```python
from build123d import *

# Parameters (mm, degrees)
F0_W            = 304.8
F0_H            = 203.2
F1_DEPTH        = 19.05
F2_W            = 228.6
F2_H            = 25.4
F3_DEPTH        = 19.051
F5_D            = 6.35
F6_R            = 6.35
F8_D            = 12.7
F9_R            = 5.4271203762
F9_R_2          = 6.35
F10_DEPTH       = 12.7
F12_D           = 9.525
F12_CBORE_D     = 15.875
F12_CBORE_DEPTH = 12.7
F13_SIZE        = 50.8


with BuildPart() as f1:
    # F0 (on Front) → F1 (new body)
    with BuildSketch(Plane.XZ):
        with Locations((152.4, 101.6)):
            Rectangle(F0_W, F0_H)
    extrude(amount=F1_DEPTH)

    # F2 (on face) → F3 (cut, through all)
    with BuildSketch(Plane.XZ.offset(19.05)):
        with Locations((152.4, 12.7)):
            Rectangle(F2_W, F2_H)
    extrude(amount=-F3_DEPTH, mode=Mode.SUBTRACT)

    # F5 (through all)
    with Locations(Plane.XZ.offset(19.05)):
        with Locations((120.65, 38.1), (184.15, 38.1)):
            Hole(F5_D / 2)

    # F6
    f6_edges = [f1.edges().sort_by_distance(p)[0] for p in [
        (38.1, -9.525, 0),
        (38.1, -9.525, 25.4),
        (0, -9.525, 0),
        (266.7, -9.525, 25.4),
        (266.7, -9.525, 0),
        (304.8, -9.525, 0),
    ]]
    fillet(f6_edges, radius=F6_R)

    # F8 (through all)
    with Locations(Plane.XZ.offset(19.05)):
        with Locations((152.4, 105.6132)):
            Hole(F8_D / 2)

    # F9 (on face) → F10 (cut)
    with BuildSketch(Plane(origin=(0, 0, 0), x_dir=(-1, 0, 0), z_dir=(0, 1, 0))):
        with Locations((-25.4, 137.3632)):
            Circle(F9_R)
        with Locations((-279.4, 137.3632)):
            Circle(F9_R_2)
    extrude(amount=-F10_DEPTH, mode=Mode.SUBTRACT)

    # F12 (through all)
    with Locations(Plane(origin=(0, 0, 0), x_dir=(-1, 0, 0), z_dir=(0, 1, 0))):
        with Locations((-286.227653817, 94.6363272378), (-285.75, 18.4363272378), (-19.05, 18.4363272378), (-16.3299310523, 94.6363272378)):
            CounterBoreHole(F12_D / 2, F12_CBORE_D / 2, F12_CBORE_DEPTH)

    # F13
    f13_edges = [f1.edges().sort_by_distance(p)[0] for p in [
        (304.8, -9.525, 203.2),
        (0, -9.525, 203.2),
    ]]
    chamfer(f13_edges, length=F13_SIZE)


solid = f1.part
```
Part model, mm, in its own coordinate system. A direction names the side the tool comes from. Round coordinates to 2 decimals unless told otherwise and drop trailing zeros. Order: outer loops, then holes, each group sorted by start corner. A loop starts at its lowest first (then second) coordinate and runs counter-clockwise, first axis right, second up. Notation, with made-up numbers: M 79.25,79.5 L 131.25,79.5 A9 cw 131.25,96.5 Z; hole C 82,53.5 d7. An arc over 180 degrees is marked long. Answer in a Markdown table with one row per item. Add a question column.
Q1. Pin check, flat tips, straight feed: pin 1 (1 mm diameter, centred on x = 271.5, y = -9, fed in from +Z); pin 2 (12.5 mm diameter, centred on x = 19.05, z = 18.44, fed in from +Y); pin 3 (2 mm diameter, centred on x = 263, y = -4, fed in from +Z). Stop position of each tip, or through.
Q2. Cut at B-B on x = 120.65. Give the cut face in (y, z) (3 decimals).
Q3. Mould opens along Z. For faces 4 (the face through (19, -12.7, 13)), 5 (the face through (288.79, -15.92, 98.65)), 6 (the face through (304.8, -9, 78)), 7 (the face through (151, -10, 25.4)) say: +Z half, -Z half, draft (parallel to the pull), parting line (faces both ways), or undercut.
Q4. Wall check: L1, parallel to X at y = -4.75, z = 90; L2, parallel to Y at x = 290, z = 88; L3, parallel to Z at x = 70, y = -13.75. Give the ranges that are in metal, low to high. Write a range as from..to.
Q5. Cut at A-A on z = 38.1. Give the cut face in (x, y) (3 decimals), and give its area (3 significant figures).
Q6. Cut at C-C on y = -9.5. Give the number of separate pieces and of enclosed holes in the cut face, and give its area (3 significant figures).
Q7. 3-axis set-ups, long thin cutter, end or side, ignore diameter. For faces 1 (the face through (150, 0, 126)), 2 (the face through (279, -12.7, 137)), 3 (the face through (264.79, -9.39, 23.59)): which of +Z, -Z, +X, -X, +Y, -Y reach the whole face in a straight line?
Q8. Cut at D-D on x = 78.5. Give the cut face in (y, z).
Established:
| question | item | result |
|---|---|---|
| 1 | pin 1 | stops at z = 186.2 |
| 1 | pin 2 | stops at y = -12.7 |
| 1 | pin 3 | stops at z = 195.2 |
| 2 | outline | M -19.05,25.4 L 0,25.4 L 0,34.925 L -19.05,34.925 Z; M -19.05,41.275 L 0,41.275 L 0,203.2 L -19.05,203.2 Z |
| 3 | face 4 | undercut |
| 3 | face 5 | undercut |
| 3 | face 6 | draft |
| 3 | face 7 | -Z half |
| 4 | L1 | x = 0..9.89, 22.77..279.78, 292.67..304.8 |
| 4 | L2 | y = -19.05..-12.7 |
| 4 | L3 | z = 25.4..203.2 |
| 5 | outline | M 0,-19.05 L 117.475,-19.05 L 117.475,0 L 0,0 Z; M 123.825,-19.05 L 180.975,-19.05 L 180.975,0 L 123.825,0 Z; M 187.325,-19.05 L 304.8,-19.05 L 304.8,0 L 187.325,0 Z |
| 5 | area | 5,560 mm2 |
| 6 | separate pieces | 1 |
| 6 | enclosed holes | 9 |
| 6 | area | 52,300 mm2 |
| 7 | face 1 | +Z, -Z, +X, -X, +Y |
| 7 | face 2 | +Y |
| 7 | face 3 | -Z, +Y, -Y |
| 8 | outline | M -19.05,25.4 L 0,25.4 L 0,203.2 L -19.05,203.2 Z |
